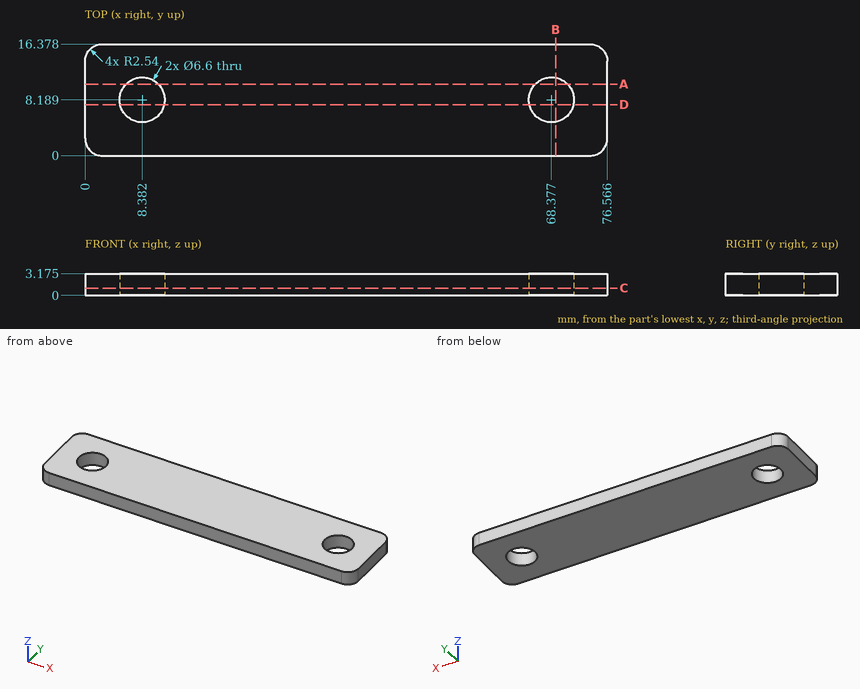
Geometry: see drawing. Coordinates: mm, zero at the bounding-box minimum. Give positions to 0.01 mm unless a question says otherwise; leave off trailing zeros. Write each loop counter-clockwise with the first axis right and the second up, starting at its lowest first coordinate (ties: lowest second). Pieces come first, ordered by that corner, then holes. Notation, with made-up numbers: (-24.75, 32.25) - (28.25, 32.25) arc R19 cw to (28.25, 65.25) - close; hole circle Ø3 at (7, -7). An arc over 180 degrees is marked (long way). Return JSON: item names as keys, results as strings. Group by question number.
1) Section A-A on y = 10.5. Return the cut outline in (x, z) (1 decimal).
2) Section B-B on x = 69. Return the cut outline in (y, z) (1 decimal).
3) Line query: line 1 (X direction, y = 8.25, z = 1.2); line 2 (X direction, y = 6.5, z = 0.2) (1 decimal); line 3 (Y direction, x = 68.5, z = 2). Output: solid intervals per line, ascending.
4) Section D-D on y = 7.5. Return the cut outline in (x, z) (1 decimal), plus the area to 3 significant figures.
5) Section C-C on z = 1.05. Return the cut outline in (x, y).
Filled in:
{
 "1": {"outline": "(0, 0) - (6, 0) - (6, 3.2) - (0, 3.2) - close; (10.7, 0) - (66, 0) - (66, 3.2) - (10.7, 3.2) - close; (70.7, 0) - (76.6, 0) - (76.6, 3.2) - (70.7, 3.2) - close"},
 "2": {"outline": "(0, 0) - (4.9, 0) - (4.9, 3.2) - (0, 3.2) - close; (11.4, 0) - (16.4, 0) - (16.4, 3.2) - (11.4, 3.2) - close"},
 "3": {"line 1": "x = 0 to 5.08, 11.68 to 65.08, 71.68 to 76.57", "line 2": "x = 0 to 5.5, 11.2 to 65.5, 71.2 to 76.6", "line 3": "y = 0 to 4.89, 11.49 to 16.38"},
 "4": {"outline": "(0, 0) - (5.2, 0) - (5.2, 3.2) - (0, 3.2) - close; (11.6, 0) - (65.1, 0) - (65.1, 3.2) - (11.6, 3.2) - close; (71.6, 0) - (76.6, 0) - (76.6, 3.2) - (71.6, 3.2) - close", "area": "202 mm^2"},
 "5": {"outline": "(0, 2.54) arc R2.54 ccw to (2.54, 0) - (74.03, 0) arc R2.54 ccw to (76.57, 2.54) - (76.57, 13.84) arc R2.54 ccw to (74.03, 16.38) - (2.54, 16.38) arc R2.54 ccw to (0, 13.84) - close; hole circle Ø6.6 at (8.38, 8.19); hole circle Ø6.6 at (68.38, 8.19)"}
}
